```python
from build123d import *

# Parameters (mm, degrees)
PAD_DEPTH              = 50
PAD001_DEPTH           = 50
SKETCH002_R            = 6
POCKET_DEPTH           = 30
SKETCH015_R            = 6
POCKET005_DEPTH        = 354.1406188228
LINEARPATTERN003_COUNT = 4
LINEARPATTERN003_PITCH = 200
CHAMFER_SIZE           = 5


with BuildPart() as part:
    # Sketch → Pad (new body)
    with BuildSketch(Plane.XY):
        with BuildLine():
            Line((-547.6857118143, 425), (19.5015988359, 27.8511695058))
            ThreePointArc((34, 0), (30.1583683281, 15.69945285), (19.5015988359, 27.8511695058))
            Line((40, 0), (34, 0))
            ThreePointArc((40, 0), (35.4804333271, 18.4699445294), (22.943057454, 32.7660817716))
            Line((22.943057454, 32.7660817716), (-544.2442531962, 429.9149122657))
            Line((-544.2442531962, 429.9149122657), (-547.6857118143, 425))
        make_face()
    extrude(amount=PAD_DEPTH)

    # Sketch001 → Pad001 (join)
    with BuildSketch(Plane.XY):
        Polygon((-94.6057566753, 107.75), (-103.1746447158, 113.75), (-1.7405688034, 113.75), (-1.7405688034, 107.75), align=None)
        Polygon((-113.171680763, 120.75), (-121.7405688034, 126.75), (-1.7405688034, 126.75), (-1.7405688034, 120.75), align=None)
    extrude(amount=PAD001_DEPTH)

    # Sketch002 → Pocket (cut)
    with BuildSketch(Plane(origin=(0, 126.75, 0), x_dir=(-1, 0, 0), z_dir=(0, 1, 0))):
        with Locations((26.7405688034, 25.24131)):
            Circle(SKETCH002_R)
    extrude(amount=-POCKET_DEPTH, mode=Mode.SUBTRACT)

    # Sketch015 (on Face2 of LinearPattern) → Pocket005 (cut, through all)
    with BuildSketch(Plane(origin=(22.943057454, 32.7660817716, 0), x_dir=(-0.8191520443, 0.5735764364, 0), z_dir=(0.5735764364, 0.8191520443, 0))):
        with Locations((663.8389678693, 25)):
            Circle(SKETCH015_R)
    pocket005 = extrude(amount=-POCKET005_DEPTH, mode=Mode.SUBTRACT)

    # LinearPattern003: Pocket005 ×4
    with Locations(*[Vector(0.8191520443, -0.5735764364, 0) * (i * LINEARPATTERN003_PITCH) for i in range(1, LINEARPATTERN003_COUNT)]):
        add(pocket005, mode=Mode.SUBTRACT)

    # Chamfer
    chamfer_edges = [part.edges().sort_by_distance(p)[0] for p in [
        (-1.740569, 123.75, 50),
        (-1.740569, 123.75, 0),
        (-1.740569, 110.75, 0),
        (-1.740569, 110.75, 50),
    ]]
    chamfer(chamfer_edges, length=CHAMFER_SIZE)


solid = part.part
```
Check sheet for the modelled part. Datum: model origin and axes. Units: mm. A direction names the side the tool comes from. Round coordinates to 2 decimals unless told otherwise and drop trailing zeros. Write each loop counter-clockwise with the first axis right and the second up, starting at its lowest first coordinate (ties: lowest second). Pieces come first, ordered by that corner, then holes. Notation, with made-up numbers: (42.25, 30.25) -> (65.25, 30.25) arc R15 ccw to (65.25, 35.25) -> close; hole circle Ø3 at (13, 83). An arc over 180 degrees is marked (long way). Put each result on its own line as item: value.
(1) Tool access check on faces 5 (the face through (-35.588, 70.139, 22.702)), 6 (the face through (-52, 120.75, 25)), 7 (the face through (-22.32, 123.79, 29.3)). Record the directions out of +Z, -Z, +X, -X, +Y, -Y that give a thin tool (end or side, any length) a straight path to the whole face; none if there is none.
Values found:
face 5: none
face 6: +Z, -Z, +X
face 7: +Y
(2) Sectioned sample at A-A (x = -442.5). Enter the section's corners in (y, z), plus the area to 3 significant figures.
Values found:
outline: (351.35, 0) -> (358.67, 0) -> (358.67, 50) -> (351.35, 50) -> close
area: 366 mm^2
(3) Go/stop test with flat-tipped pins: pin 1 Ø11 at (x, z) = (-26.74, 25.24) entering from -Y; pin 2 Ø10 at (x, z) = (-126.5, 21) entering from -Y; pin 3 Ø12 at (x, z) = (-424.5, 25) entering from +Y. Record where each tip stops, or that it passes through.
Values found:
pin 1: stops at y = 56.38
pin 2: stops at y = 126.58
pin 3: stops at y = 350.27
(4) Sectioned sample at B-B (y = 283). Enter the section's corners in (x, z).
Values found:
outline: (-344.89, 0) -> (-334.43, 0) -> (-334.43, 50) -> (-344.89, 50) -> close
(5) Material ranges on line 1 (Y direction, x = -79, z = 31.5); line 2 (X direction, y = 188.5, z = 32.5); line 3 (X direction, y = 57, z = 21.5), recorded low to high.
Values found:
line 1: y = 96.82 to 104.15, 107.75 to 113.75, 120.75 to 126.75
line 2: x = -209.93 to -199.47
line 3: x = -22.13 to -11.67
(6) Mould release check, pull along Y, two halves, no side actions. Record for faces 1 (the face through (-29.85, 69.73, 13.54)), 2 (the face through (-48, 113.75, 25)), 3 (the face through (-22.32, 110.79, 29.3)), 4 (the face through (-57, 126.75, 25)): released by +Y, released by -Y, zero draft, split by the parting line, or undercut.
Values found:
face 1: undercut
face 2: undercut
face 3: zero draft
face 4: released by +Y
